```python
from build123d import *

# Parameters (mm, degrees)
IZIM1_W               = 50
IZIM1_H               = 100
TABAN_FLAN_1_DEPTH    = 10
KES_EKSTR_ZYON1_DEPTH = 20
RADYUS1_R             = 5
IZIM7_R               = 15
KES_EKSTR_ZYON2_DEPTH = 10
RADYUS2_R             = 3


# Sheet-metal steps are written as plain solids
with BuildPart() as part:
    # Çizim1 → Taban-Flanş1 (new body)
    with BuildSketch(Plane.XY):
        Rectangle(IZIM1_W, IZIM1_H)
    extrude(amount=-TABAN_FLAN_1_DEPTH)

    # Çizim6 → Kes-Ekstrüzyon1 (cut)
    with BuildSketch(Plane.XY):
        with BuildLine():
            Line((5.5, 22.5), (5.5, 7.5))
            ThreePointArc((5.5, 7.5), (0, 2), (-5.5, 7.5))
            Line((-5.5, 7.5), (-5.5, 22.5))
            ThreePointArc((-5.5, 22.5), (0, 28), (5.5, 22.5))
        make_face()
        with BuildLine():
            Line((-5.5, -37.5), (-5.5, -22.5))
            ThreePointArc((-5.5, -22.5), (0, -17), (5.5, -22.5))
            Line((5.5, -22.5), (5.5, -37.5))
            ThreePointArc((5.5, -37.5), (0, -43), (-5.5, -37.5))
        make_face()
    extrude(amount=-KES_EKSTR_ZYON1_DEPTH, mode=Mode.SUBTRACT)

    # Radyus1
    radyus1_edges = [part.edges().sort_by_distance(p)[0] for p in [
        (25, -50, -5),
        (-25, -50, -5),
    ]]
    fillet(radyus1_edges, radius=RADYUS1_R)

    # Çizim7 → Kes-Ekstrüzyon2 (cut)
    with BuildSketch(Plane.XY):
        with Locations((0, 51)):
            Circle(IZIM7_R)
    extrude(amount=-KES_EKSTR_ZYON2_DEPTH, mode=Mode.SUBTRACT)

    # Radyus2
    radyus2_edges = [part.edges().sort_by_distance(p)[0] for p in [
        (-14.966629547, 50, -5),
        (14.966629547, 50, -5),
        (-25, 50, -5),
        (25, 50, -5),
    ]]
    fillet(radyus2_edges, radius=RADYUS2_R)


solid = part.part
```
Check sheet for the modelled part. Datum: model origin and axes. Units: mm. A direction names the side the tool comes from. Coordinates: 2 decimals unless noted, no trailing zeros. Order: outer loops, then holes, each group sorted by start corner. A loop starts at its lowest first (then second) coordinate and runs counter-clockwise, first axis right, second up. Notation, with made-up numbers: (29.5, 73.5) -> (37.5, 73.5) arc R23 ccw to (37.5, 104.5) -> close; hole circle Ø8 at (70.5, 51). An arc over 180 degrees is marked (long way). Write item = value, one per line. Start each with the question number.
1) Material ranges on L1, parallel to Y at x = 0.5, z = -7.75; L2, parallel to X at y = -35, z = -2.5; L3, parallel to Y at x = 4.5, z = -2.5, recorded low to high.
2) Mould release check, pull along X, two halves, no side actions. Record for faces 1 (the flat face through (25, 0, -5)), 2 (the cylindrical face through (-24.14, 49.1, -5.07)), 3 (the flat face through (5.5, -30, -5)), 4 (the flat face through (0, 1, 0)): +X half, -X half, draft (parallel to the pull), parting line (faces both ways), or undercut.
3) Access from +Z, -Z, +X, -X, +Y, -Y to the whole of each face (thin tool, end or side, straight path). Record for faces 5 (the flat face through (-5.5, -30, -5)), 6 (the cylindrical face through (15.66, 49.33, -4.93)), 7 (the flat face through (-25, 0, -5)).
4) Cross-section at A-A (y = -34.5). Enter the section's corners in (x, z), then the cut area to 3 significant figures.
5) Cross-section at B-B (z = -7). Enter the section's corners in (x, y), then the cut area to 3 significant figures.
6) Go/stop test with flat-tipped pins: P1, Ø1, axis at x = 3.5, z = -6, coming from the +Y side; P2, Ø4, axis at x = 3, z = -7.5, coming from the +Y side; P3, Ø6, axis at x = -1, y = -24.5, coming from the +Z side. Record where each tip stops, or that it passes through.
7) Cross-section at C-C (x = 0). Enter the section's corners in (y, z).
Ans:
q1.L1 = -50 to -42.98, -17.02 to 2.02, 27.98 to 36.01
q1.L2 = -25 to -5.5, 5.5 to 25
q1.L3 = -50 to -40.66, -19.34 to 4.34, 25.66 to 36.69
q2.face_1 = +X half
q2.face_2 = -X half
q2.face_3 = undercut
q2.face_4 = draft
q3.face_5 = +Z, -Z
q3.face_6 = +Z, -Z, +Y
q3.face_7 = +Z, -Z, -X, +Y, -Y
q4.outline = (-25, -10) -> (-5.5, -10) -> (-5.5, 0) -> (-25, 0) -> close; (5.5, -10) -> (25, -10) -> (25, 0) -> (5.5, 0) -> close
q4.area = 390 mm²
q5.outline = (-25, -45) arc R5 ccw to (-20, -50) -> (20, -50) arc R5 ccw to (25, -45) -> (25, 47) arc R3 ccw to (22, 50) -> (17.55, 50) arc R3 ccw to (14.62, 47.67) arc R15 cw to (-14.62, 47.67) arc R3 ccw to (-17.55, 50) -> (-22, 50) arc R3 ccw to (-25, 47) -> close; hole (-5.5, -37.5) arc R5.5 ccw to (5.5, -37.5) -> (5.5, -22.5) arc R5.5 ccw to (-5.5, -22.5) -> close; hole (-5.5, 7.5) arc R5.5 ccw to (5.5, 7.5) -> (5.5, 22.5) arc R5.5 ccw to (-5.5, 22.5) -> close
q5.area = 4,140 mm²
q6.P1 = 36.54
q6.P2 = 36.86
q6.P3 = through
q7.outline = (-50, -10) -> (-43, -10) -> (-43, 0) -> (-50, 0) -> close; (-17, -10) -> (2, -10) -> (2, 0) -> (-17, 0) -> close; (28, -10) -> (36, -10) -> (36, 0) -> (28, 0) -> close
